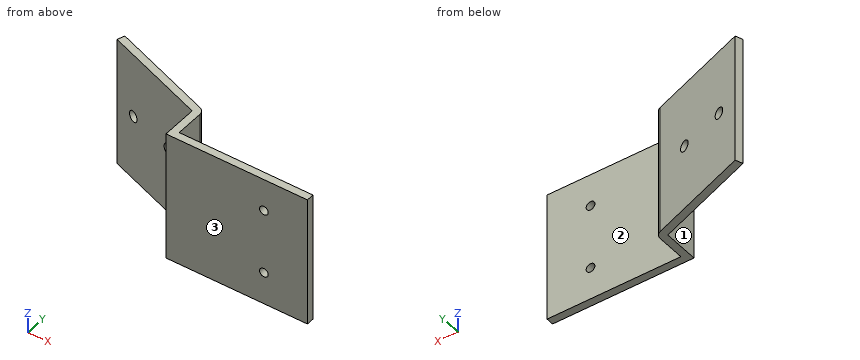
from build123d import *

# Parameters (mm, degrees)
SKETCH1_W           = 65
SKETCH1_H           = 60
BOSS_EXTRUDE1_DEPTH = 3.5
SKETCH2_W           = 3.5
SKETCH2_H           = 60
BOSS_EXTRUDE2_DEPTH = 13
BOSS_EXTRUDE5_DEPTH = 60
SKETCH9_R           = 2
CUT_EXTRUDE1_DEPTH  = 60
SKETCH10_R          = 2.5
CUT_EXTRUDE2_DEPTH  = 60


with BuildPart() as part:
    # Sketch1 → Boss-Extrude1 (new body)
    with BuildSketch(Plane(origin=(0, 0, 0), x_dir=(1, 0, 0), z_dir=(0, 1, 0))):
        with Locations((32.5, -30)):
            Rectangle(SKETCH1_W, SKETCH1_H)
    extrude(amount=BOSS_EXTRUDE1_DEPTH)

    # Sketch2 → Boss-Extrude2 (add)
    with BuildSketch(Plane(origin=(0, 3.5, 0), x_dir=(1, 0, 0), z_dir=(0, 1, 0))):
        with Locations((1.75, -30)):
            Rectangle(SKETCH2_W, SKETCH2_H)
    extrude(amount=BOSS_EXTRUDE2_DEPTH)

    # Sketch7 → Boss-Extrude5 (add)
    with BuildSketch(Plane.XY.offset(60)):
        with BuildLine():
            Line((0, 16.5), (-46.984631039, 33.601007166))
            Line((-46.984631039, 33.601007166), (-45.787560538, 36.889931339))
            Line((-45.787560538, 36.889931339), (1.197070502, 19.788924173))
            ThreePointArc((1.197070502, 19.788924173), (2.867032155, 18.507517527), (3.5, 16.5))
            Line((3.5, 16.5), (3.5, 3.5))
            Line((3.5, 3.5), (65, 3.5))
            Line((65, 3.5), (65, 0))
            Line((65, 0), (0, 0))
            Line((0, 0), (0, 16.5))
        make_face()
    extrude(amount=-BOSS_EXTRUDE5_DEPTH)

    # Sketch9 → Cut-Extrude1 (cut)
    with BuildSketch(Plane(origin=(0, 3.5, 0), x_dir=(1, 0, 0), z_dir=(0, 1, 0))):
        with Locations((45, -15)):
            Circle(SKETCH9_R)
        with Locations((45, -45)):
            Circle(SKETCH9_R)
    extrude(amount=-CUT_EXTRUDE1_DEPTH, mode=Mode.SUBTRACT)

    # Sketch10 → Cut-Extrude2 (cut)
    with BuildSketch(Plane(origin=(6.500068282, 17.858790828, 0), x_dir=(0.939692621, -0.342020143, 0), z_dir=(0.342020143, 0.939692621, 0))):
        with Locations((-44.839233595, -30.181228876)):
            Circle(SKETCH10_R)
        with Locations((-21.839233595, -30.181228876)):
            Circle(SKETCH10_R)
    extrude(amount=-CUT_EXTRUDE2_DEPTH, mode=Mode.SUBTRACT)


solid = part.part
Geometry check sheet. Reference: the model listing, model coordinates, mm. Face numbers are marked on the shaded views. A direction names the side the tool comes from. Round coordinates to 2 decimals unless told otherwise and drop trailing zeros. Loops run counter-clockwise (first coordinate to the right, second up) from the corner with the lowest first, then second, coordinate; pieces in that order, holes last. Notation, with made-up numbers: (-20.75, -36) - (16.25, -36) arc R18 ccw to (16.25, -13) - close; hole circle Ø2 at (36, 17). An arc over 180 degrees is marked (long way). Answer as CSV lines item,"result".
(1) Cross-section at B-B, the plane z = 15. Enter the section's corners in (x, y), and give its area (3 significant figures).
Output values:
outline,"(-46.98, 33.6) - (0, 16.5) - (0, 0) - (43, 0) - (43, 3.5) - (3.5, 3.5) - (3.5, 16.5) arc R3.5 ccw to (1.2, 19.79) - (-45.79, 36.89) - close; (47, 0) - (65, 0) - (65, 3.5) - (47, 3.5) - close"
area,"441 mm²"
(2) Material ranges on line 1 along Z through (x, y) = (45, 2); line 2 along X through (y, z) = (0.7, 45); line 3 along Y through (x, z) = (17, 32), recorded low to high.
Output values:
line 1,"z = 0 to 13, 17 to 43, 47 to 60"
line 2,"x = 0 to 43, 47 to 65"
line 3,"y = 0 to 3.5"
(3) Set-up check for the marked faces 1, 2 and 3: record each of +Z, -Z, +X, -X, +Y, -Y from which the full face is reachable in a straight line by a thin tool's end or side.
Output values:
face 1,"+Z, -Z, -X, -Y"
face 2,"+Z, -Z, +X, +Y"
face 3,"+Z, -Z, +X, -X, -Y"
(4) Cross-section at D-D, the plane x = 33. Enter the section's corners in (y, z), and give its area (3 significant figures).
Output values:
outline,"(0, 0) - (3.5, 0) - (3.5, 60) - (0, 60) - close"
area,"210 mm²"
(5) Cross-section at A-A, the plane x = 45. Enter the section's corners in (y, z).
Output values:
outline,"(0, 0) - (3.5, 0) - (3.5, 13) - (0, 13) - close; (0, 17) - (3.5, 17) - (3.5, 43) - (0, 43) - close; (0, 47) - (3.5, 47) - (3.5, 60) - (0, 60) - close"
(6) Cross-section at C-C, the plane z = 4. Enter the section's corners in (x, y).
Output values:
outline,"(-46.98, 33.6) - (0, 16.5) - (0, 0) - (65, 0) - (65, 3.5) - (3.5, 3.5) - (3.5, 16.5) arc R3.5 ccw to (1.2, 19.79) - (-45.79, 36.89) - close"
(7) Depth check by flat-ended pin: pin 1 Ø1.5 at (x, z) = (-5.5, 26) entering from -Y; pin 2 Ø8 at (y, z) = (17.5, 43) entering from +X; pin 3 Ø12 at (y, z) = (8.5, 12.5) entering from -X. Enter the tip coordinate at first touch or a pass-through.
Output values:
pin 1,"stops at y = 18.23"
pin 2,"stops at x = 3.5"
pin 3,"stops at x = 0"
